```python
from build123d import *

# Parameters (mm, degrees)
SKETCH1_R           = 17.5
BOSS_EXTRUDE1_DEPTH = 8
SKETCH5_R           = 16.5
CUT_EXTRUDE2_DEPTH  = 1
SKETCH11_R          = 1.67
CUT_EXTRUDE5_DEPTH  = 1.15
CIRPATTERN1_COUNT   = 4
SKETCH13_W          = 18
SKETCH13_H          = 18
SKETCH13_W_2        = 16.9
SKETCH13_H_2        = 16.9
BOSS_EXTRUDE3_DEPTH = 1.3
SKETCH12_W          = 18
SKETCH12_H          = 18
BOSS_EXTRUDE2_DEPTH = 0.8
CUT_EXTRUDE6_DEPTH  = 27.266708968


with BuildPart() as part:
    # Sketch1 → Boss-Extrude1 (new body)
    with BuildSketch(Plane(origin=(0, 0, 0), x_dir=(1, 0, 0), z_dir=(0, 1, 0))):
        with Locations(Location((0, 0, 0), (0, 0, 270))):
            Circle(SKETCH1_R)
    extrude(amount=BOSS_EXTRUDE1_DEPTH)

    # Sketch5 → Cut-Extrude2 (cut)
    with BuildSketch(Plane.XZ):
        with Locations(Location((0, 0, 0), (0, 0, 270))):
            Circle(SKETCH5_R)
    extrude(amount=-CUT_EXTRUDE2_DEPTH, mode=Mode.SUBTRACT)

    # Sketch11 → Cut-Extrude5 (cut)
    with BuildSketch(Plane(origin=(0, 8, 0), x_dir=(1, 0, 0), z_dir=(0, 1, 0))):
        with Locations(Location((0.106708516, 14.783412681, 0), (0, 0, 270))):
            Circle(SKETCH11_R)
    cut_extrude5 = extrude(amount=-CUT_EXTRUDE5_DEPTH, mode=Mode.SUBTRACT)

    # CirPattern1: Cut-Extrude5 ×4 about axis
    cirpattern1_axis = Axis((0, 0, 0), (0, 1, 0))
    for i in range(1, CIRPATTERN1_COUNT):
        add(cut_extrude5.rotate(cirpattern1_axis, i * 360 / CIRPATTERN1_COUNT), mode=Mode.SUBTRACT)

    # Sketch13 → Boss-Extrude3 (add)
    with BuildSketch(Plane(origin=(0, 8, 0), x_dir=(1, 0, 0), z_dir=(0, 1, 0))):
        Rectangle(SKETCH13_W, SKETCH13_H)
        Rectangle(SKETCH13_W_2, SKETCH13_H_2, mode=Mode.SUBTRACT)
    extrude(amount=BOSS_EXTRUDE3_DEPTH)

    # Sketch12 → Boss-Extrude2 (add)
    with BuildSketch(Plane(origin=(0, 8, 0), x_dir=(1, 0, 0), z_dir=(0, 1, 0))):
        Rectangle(SKETCH12_W, SKETCH12_H)
    extrude(amount=BOSS_EXTRUDE2_DEPTH)

    # Sketch14 → Cut-Extrude6 (cut, through all)
    with BuildSketch(Plane(origin=(0, 8.8, 0), x_dir=(1, 0, 0), z_dir=(0, 1, 0))):
        with BuildLine():
            ThreePointArc((-7, -5.85), (-6.663172798, -6.663172798), (-5.85, -7))
            Line((-5.85, -7), (5.85, -7))
            ThreePointArc((5.85, -7), (6.663172798, -6.663172798), (7, -5.85))
            Line((7, -5.85), (7, 5.85))
            ThreePointArc((7, 5.85), (6.663172798, 6.663172798), (5.85, 7))
            Line((5.85, 7), (-5.85, 7))
            ThreePointArc((-5.85, 7), (-6.663172798, 6.663172798), (-7, 5.85))
            Line((-7, 5.85), (-7, -5.85))
        make_face()
    extrude(amount=-CUT_EXTRUDE6_DEPTH, mode=Mode.SUBTRACT)


solid = part.part
```
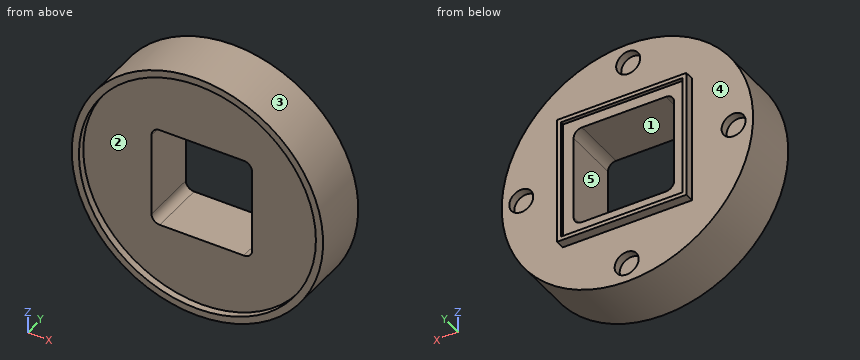
Geometry: final body of the model. Coordinates: model frame, mm. Face numbers are marked on the shaded views. A direction names the side the tool comes from. Coordinates: 2 decimals unless noted, no trailing zeros. Write each loop counter-clockwise with the first axis right and the second up, starting at its lowest first coordinate (ties: lowest second). Pieces come first, ordered by that corner, then holes. Notation, with made-up numbers: M 56,65 L 105,65 A25 cw 105,77 Z; hole C 10,46 d6. An arc over 180 degrees is marked long. Answer as CSV lines item,"result". Start each with the question number.
Q1. Cut plane A-A on y = 2.75. Return the cut outline in (x, z), then the cut area to 3 significant figures.
Q2. Cut plane D-D on x = 3.5. Return the cut outline in (y, z), then the cut area to 3 significant figures.
Q3. Mould query, pull axis X, two halves, no side actions, for the marked faces 3, 4 and 5. Classes: released by +X, released by -X, zero draft, split by the parting line, or undercut.
Q4. Cut plane C-C on z = -4.5. Return the cut outline in (x, y).
Q5. Cut plane B-B on x = -1. Return the cut outline in (y, z), then the cut area to 3 significant figures.
Q6. Pin query (flat end, axial travel): P1, Ø1.4, axis at y = 8.5, z = -2, coming from the -X side; P2, Ø10, axis at x = 6.5, z = -4.5, coming from the -Y side; P3, Ø2, axis at x = 10.5, y = 2, coming from the +Z side. Return the tip coordinate at first contact, or that it passes through.
Q7. Reachability of the marked faces 1 and 2 from +Z, -Z, +X, -X, +Y, -Y: full face, straight path, thin tool, end or side. Return the list, or none.
Q8. Line query: line 1 (X direction, y = 4, z = 0.5); line 2 (Y direction, x = -5, z = -8.5); line 3 (Y direction, x = 3, z = 8). Output: solid intervals per line, ascending. Write a range as from..to.
Findings below:
1,outline,"C 0,0 d35; hole M -7,-5.85 A1.15 ccw -5.85,-7 L 5.85,-7 A1.15 ccw 7,-5.85 L 7,5.85 A1.15 ccw 5.85,7 L -5.85,7 A1.15 ccw -7,5.85 Z"
1,area,"767 mm2"
2,outline,"M 0,-17.15 L 8,-17.15 L 8,-9 L 9.3,-9 L 9.3,-8.45 L 8.8,-8.45 L 8.8,-7 L 1,-7 L 1,-16.12 L 0,-16.12 Z; M 0,16.12 L 1,16.12 L 1,7 L 8.8,7 L 8.8,8.45 L 9.3,8.45 L 9.3,9 L 8,9 L 8,17.15 L 0,17.15 Z"
2,area,"148 mm2"
3,face 3,"split by the parting line"
3,face 4,"zero draft"
3,face 5,"undercut"
4,outline,"M -16.91,0 L -15.87,0 L -15.87,1 L -7,1 L -7,8.8 L -8.45,8.8 L -8.45,9.3 L -9,9.3 L -9,8 L -16.91,8 Z; M 7,1 L 15.87,1 L 15.87,0 L 16.91,0 L 16.91,8 L 9,8 L 9,9.3 L 8.45,9.3 L 8.45,8.8 L 7,8.8 Z"
5,outline,"M 0,-17.47 L 8,-17.47 L 8,-16.03 L 6.85,-16.03 L 6.85,-13.53 L 8,-13.53 L 8,-9 L 9.3,-9 L 9.3,-8.45 L 8.8,-8.45 L 8.8,-7 L 1,-7 L 1,-16.47 L 0,-16.47 Z; M 0,16.47 L 1,16.47 L 1,7 L 8.8,7 L 8.8,8.45 L 9.3,8.45 L 9.3,9 L 8,9 L 8,13.37 L 6.85,13.37 L 6.85,16.19 L 8,16.19 L 8,17.47 L 0,17.47 Z"
5,area,"146 mm2"
6,P1,"stops at x = -17.43"
6,P2,"stops at y = 1"
6,P3,"stops at z = 14.7"
7,face 1,"+Y, -Y"
7,face 2,"-Y"
8,line 1,"x = -17.49..-7, 7..17.49"
8,line 2,"y = 1..9.3"
8,line 3,"y = 1..8.8"
